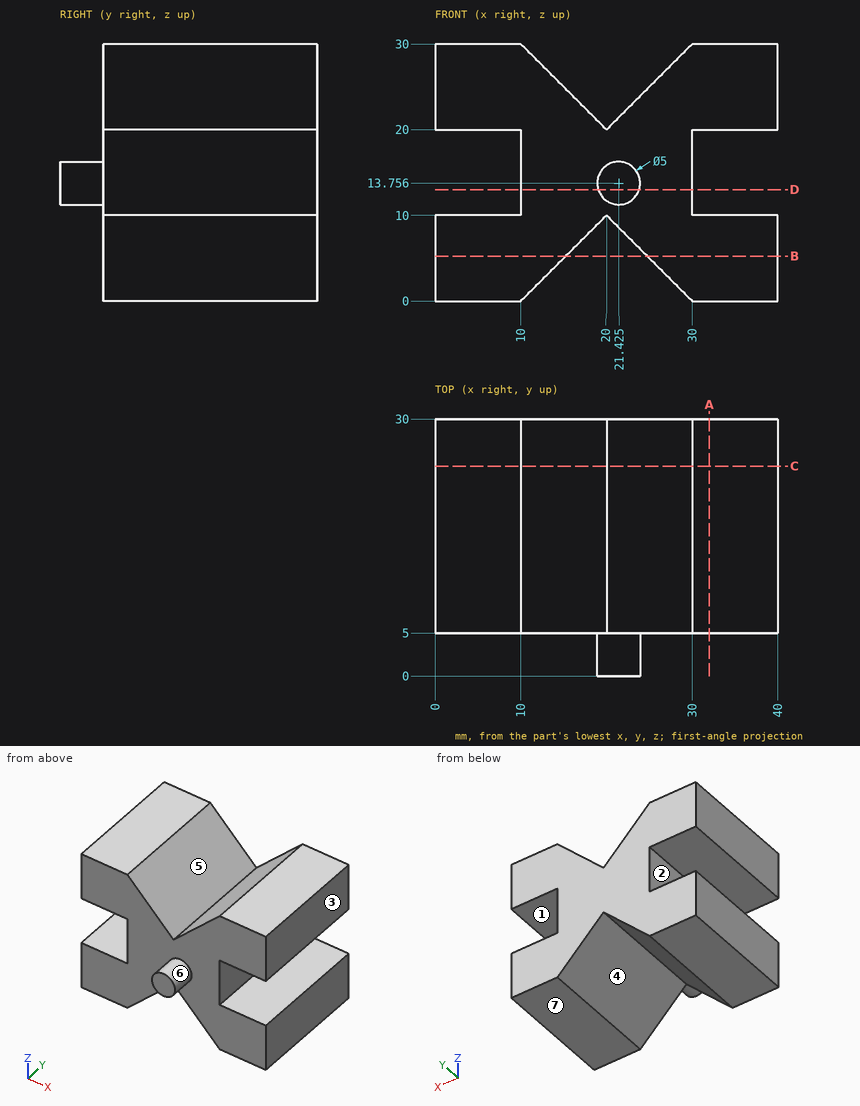
Could you check a few things on this drawing? It's one solid part, dimensions in mm from its lowest x, y, z. A direction names the side the tool comes from. Coordinates: 2 decimals unless noted, no trailing zeros. Order: outer loops, then holes, each group sorted by start corner. A loop starts at its lowest first (then second) coordinate and runs counter-clockwise, first axis right, second up.
1) Imagine slicing it at D-D on z = 13. List the corners of the cut face in (x, y) for me.
2) We'd pull the mould along X, two halves only. Please class the marked faces 4, 5, 6 and 7: +X half, -X half, draft (parallel to the pull), parting line (faces both ways), or undercut.
3) Imagine slicing it at A-A on x = 32. List the corners of the cut face in (y, z) for me.
4) Which directions (+Z, -Z, +X, -X, +Y, -Y) give clear straight access to the entire face, cutting with the end or side of a thin tool? Please do the marked faces 1, 2 and 3.
5) Will these pins go through, and if not, where does the flat tip stop? pin 1 (1.5 mm diameter, centred on y = 25, z = 20, fed in from -X); pin 2 (2 mm diameter, centred on x = 23.5, y = 23, fed in from +Z); pin 3 (10 mm diameter, centred on x = 20, y = 8.5, fed in from +Z); pin 4 (5 mm diameter, centred on y = 23.5, z = 13.5, fed in from -X).
6) Imagine slicing it at B-B on z = 5.25. List the corners of the cut face in (x, y) for me.
7) Imagine slicing it at C-C on y = 24.5. List the corners of the cut face in (x, z) for me.
8) I need wall thicknesses on line 1 (Z direction, x = 8, y = 6.25); line 2 (Y direction, x = 11, z = 25.25); line 3 (X direction, y = 10.25, z = 11.75). Which ranges of each line are inside material? Lowest first, please.
Response values:
1. outline: (10, 5) - (19.04, 5) - (19.04, 0) - (23.81, 0) - (23.81, 5) - (30, 5) - (30, 30) - (10, 30) - close
2. face 4: undercut
2. face 5: undercut
2. face 6: parting line
2. face 7: draft
3. outline: (5, 0) - (30, 0) - (30, 10) - (5, 10) - close; (5, 20) - (30, 20) - (30, 30) - (5, 30) - close
4. face 1: +X, +Y, -Y
4. face 2: -X, +Y, -Y
4. face 3: +Z, -Z, +X, +Y, -Y
5. pin 1: stops at x = 0
5. pin 2: stops at z = 24.5
5. pin 3: stops at z = 25
5. pin 4: stops at x = 10
6. outline: (0, 5) - (15.25, 5) - (15.25, 30) - (0, 30) - close; (24.75, 5) - (40, 5) - (40, 30) - (24.75, 30) - close
7. outline: (0, 0) - (10, 0) - (20, 10) - (30, 0) - (40, 0) - (40, 10) - (30, 10) - (30, 20) - (40, 20) - (40, 30) - (30, 30) - (20, 20) - (10, 30) - (0, 30) - (0, 20) - (10, 20) - (10, 10) - (0, 10) - close
8. line 1: z = 0 to 10, 20 to 30
8. line 2: y = 5 to 30
8. line 3: x = 10 to 30
